Part print with two shaded views. Sizes in mm from the minimum x, y, z corner. A direction names the side the tool comes from. Round coordinates to 2 decimals unless told otherwise and drop trailing zeros. Write each loop counter-clockwise with the first axis right and the second up, starting at its lowest first coordinate (ties: lowest second). Pieces come first, ordered by that corner, then holes.
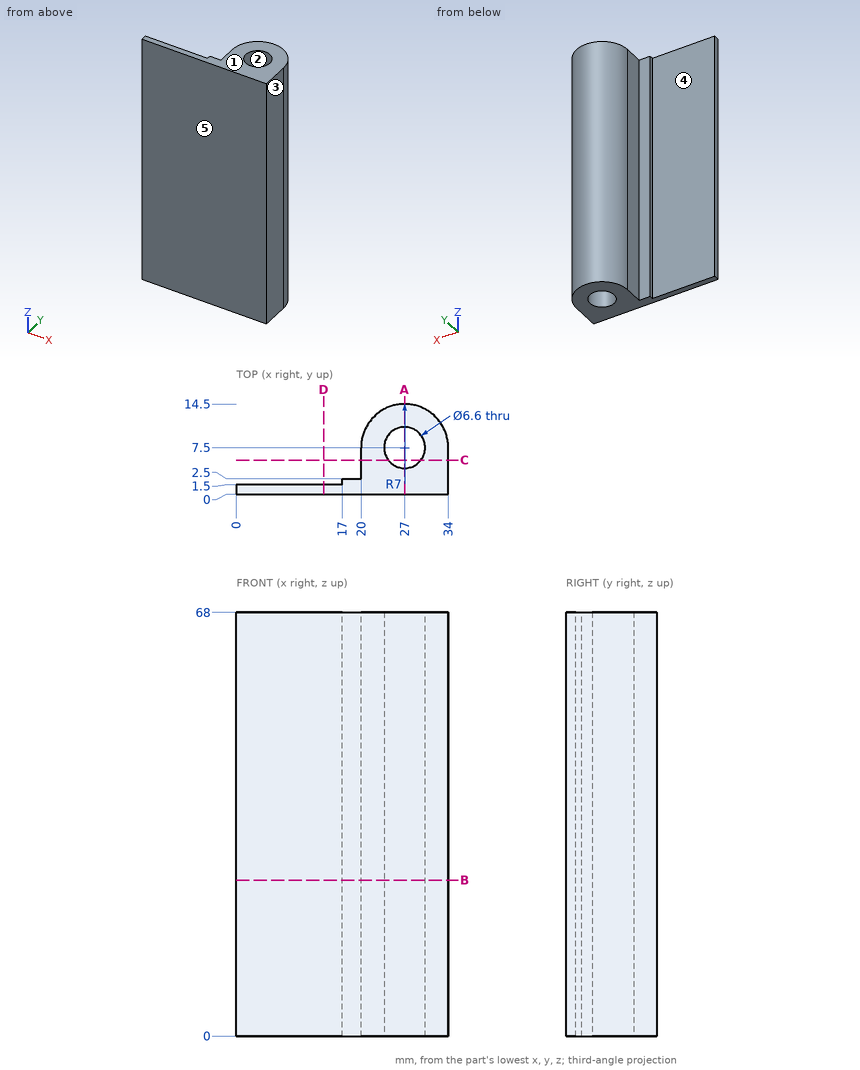
Q1. Which spindle directions (+Z, -Z, +X, -X, +Y, -Y) get a long thin tool onto all of the face, cutting with end or side? Do the marked faces 4 and 5. Say none if no direction does.
Values follow:
face 4: +Z, -Z, -X, +Y
face 5: +Z, -Z, +X, -X, -Y
Q2. Cut at D-D on x = 14. Write the cut outline in (y, z), plus the area to 3 significant figures.
Values follow:
outline: (0, 0) - (1.5, 0) - (1.5, 68) - (0, 68) - close
area: 102 mm2
Q3. Cut at C-C on y = 5.5. Write the cut outline in (x, z), plus the area to 3 significant figures.
Values follow:
outline: (20, 0) - (24.38, 0) - (24.38, 68) - (20, 68) - close; (29.62, 0) - (34, 0) - (34, 68) - (29.62, 68) - close
area: 595 mm2
Q4. Drop flat-ended pins along their axis: pin 1 (6 mm diameter, centred on y = 12.5, z = 49, fed in from -X); pin 2 (1.5 mm diameter, centred on y = 9, z = 15.5, fed in from -X); pin 3 (0.5 mm diameter, centred on y = 2, z = 39, fed in from -X); pin 4 (5 mm diameter, centred on x = 20.5, z = 57.5, fed in from -Y). Give the stop position or say it passes through.
Values follow:
pin 1: stops at x = 20.29
pin 2: stops at x = 20.04
pin 3: stops at x = 17
pin 4: stops at y = 0
Q5. Cut at B-B on z = 25. Write the cut outline in (x, y), plus the area to 3 significant figures.
Values follow:
outline: (0, 0) - (34, 0) - (34, 7.5) arc R7 ccw to (20, 7.5) - (20, 2.5) - (17, 2.5) - (17, 1.5) - (0, 1.5) - close; hole circle Ø6.6 at (27, 7.5)
area: 181 mm2
Q6. Wall check: L1, parallel to X at y = 7.25, z = 29; L2, parallel to Y at x = 27, z = 35; L3, parallel to X at y = 3.25, z = 34.5. Give the ranges that are in metal, low to high.
Values follow:
L1: x = 20 to 23.71, 30.29 to 34
L2: y = 0 to 4.2, 10.8 to 14.5
L3: x = 20 to 34
Q7. Cut at A-A on x = 27. Write the cut outline in (y, z), plus the area to 3 significant figures.
Values follow:
outline: (0, 0) - (4.2, 0) - (4.2, 68) - (0, 68) - close; (10.8, 0) - (14.5, 0) - (14.5, 68) - (10.8, 68) - close
area: 537 mm2
Q8. Mould opens along X. For the marked faces 1, 2 and 3 say: +X half, -X half, draft (parallel to the pull), parting line (faces both ways), or undercut.
Values follow:
face 1: draft
face 2: undercut
face 3: +X half
